from build123d import *

# Parameters (mm, degrees)
ESQUISSE1_W             = 110
ESQUISSE1_H             = 70
BOSS_EXTRU_1_DEPTH      = 5
ESQUISSE2_R             = 2.5
ESQUISSE2_R_2           = 1.3
ENL_V_MAT_EXTRU_1_DEPTH = 131.479883507
ESQUISSE4_R             = 2.5
ENL_V_MAT_EXTRU_2_DEPTH = 3
ENL_V_MAT_EXTRU_3_DEPTH = 131.479883507
CONG_1_R                = 10


with BuildPart() as part:
    # Esquisse1 → Boss.-Extru.1 (new body)
    with BuildSketch(Plane(origin=(0, 0, 0), x_dir=(1, 0, 0), z_dir=(0, 1, 0))):
        with Locations((55, 35)):
            Rectangle(ESQUISSE1_W, ESQUISSE1_H)
    extrude(amount=BOSS_EXTRU_1_DEPTH)

    # Esquisse2 → Enlèv. mat.-Extru.1 (cut, through all)
    with BuildSketch(Plane(origin=(0, 5, 0), x_dir=(1, 0, 0), z_dir=(0, 1, 0))):
        with Locations(Location((9, 59, 0), (0, 0, 270))):
            Circle(ESQUISSE2_R)
        with Locations(Location((9, 11, 0), (0, 0, 270))):
            Circle(ESQUISSE2_R)
        with Locations(Location((101, 11, 0), (0, 0, 270))):
            Circle(ESQUISSE2_R)
        with Locations(Location((101, 59, 0), (0, 0, 270))):
            Circle(ESQUISSE2_R)
        with Locations(Location((25, 46.176778867, 0), (0, 0, 270))):
            Circle(ESQUISSE2_R_2)
        with Locations(Location((25, 21.176778867, 0), (0, 0, 270))):
            Circle(ESQUISSE2_R_2)
        with Locations(Location((85, 21.176778867, 0), (0, 0, 270))):
            Circle(ESQUISSE2_R_2)
        with Locations(Location((85, 46.176778867, 0), (0, 0, 270))):
            Circle(ESQUISSE2_R_2)
    extrude(amount=-ENL_V_MAT_EXTRU_1_DEPTH, mode=Mode.SUBTRACT)

    # Esquisse4 → Enlèv. mat.-Extru.2 (cut)
    with BuildSketch(Plane(origin=(0, 5, 0), x_dir=(1, 0, 0), z_dir=(0, 1, 0))):
        with Locations(Location((25, 46.176778867, 0), (0, 0, 270))):
            Circle(ESQUISSE4_R)
        with Locations(Location((25, 21.176778867, 0), (0, 0, 270))):
            Circle(ESQUISSE4_R)
        with Locations(Location((85, 21.176778867, 0), (0, 0, 270))):
            Circle(ESQUISSE4_R)
        with Locations(Location((85, 46.176778867, 0), (0, 0, 270))):
            Circle(ESQUISSE4_R)
    extrude(amount=-ENL_V_MAT_EXTRU_2_DEPTH, mode=Mode.SUBTRACT)

    # Esquisse5 → Enlèv. mat.-Extru.3 (cut, through all)
    with BuildSketch(Plane(origin=(0, 5, 0), x_dir=(1, 0, 0), z_dir=(0, 1, 0))):
        with BuildLine():
            Line((35.175146904, 65), (74.824853096, 65))
            ThreePointArc((74.824853096, 65), (79.824853096, 60), (74.824853096, 55))
            Line((74.824853096, 55), (35.175146904, 55))
            ThreePointArc((35.175146904, 55), (30.175146904, 60), (35.175146904, 65))
        make_face()
        with BuildLine():
            Line((16.226090532, 40.659734035), (93.773909468, 40.659734035))
            ThreePointArc((93.773909468, 40.659734035), (99.433643503, 35), (93.773909468, 29.340265965))
            Line((93.773909468, 29.340265965), (16.226090532, 29.340265965))
            ThreePointArc((16.226090532, 29.340265965), (10.566356497, 35), (16.226090532, 40.659734035))
        make_face()
        with BuildLine():
            Line((33.566737233, 15), (76.433262767, 15))
            ThreePointArc((76.433262767, 15), (81.433262767, 10), (76.433262767, 5))
            Line((76.433262767, 5), (33.566737233, 5))
            ThreePointArc((33.566737233, 5), (28.566737233, 10), (33.566737233, 15))
        make_face()
    extrude(amount=-ENL_V_MAT_EXTRU_3_DEPTH, mode=Mode.SUBTRACT)

    # Congé1
    cong_1_edges = [part.edges().sort_by_distance(p)[0] for p in [
        (0, 2.5, -70),
        (110, 2.5, -70),
        (110, 2.5, 0),
        (0, 2.5, 0),
    ]]
    fillet(cong_1_edges, radius=CONG_1_R)


solid = part.part
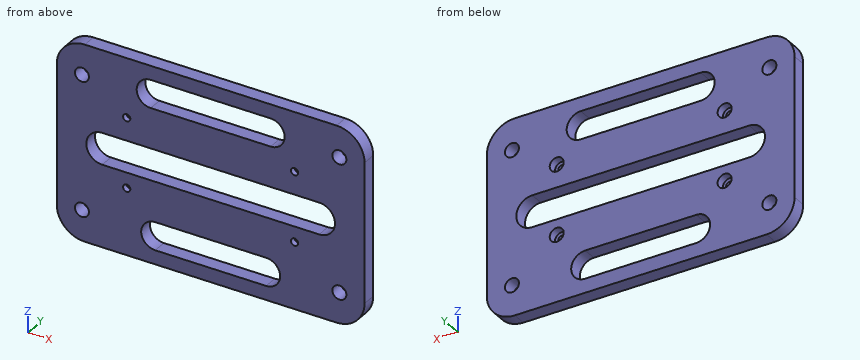
The listing builds one solid part. Answer for the finished solid, in the listing's coordinates (mm). Round coordinates to 2 decimals unless told otherwise and drop trailing zeros. Order: outer loops, then holes, each group sorted by start corner. A loop starts at its lowest first (then second) coordinate and runs counter-clockwise, first axis right, second up. Notation, with made-up numbers: (-6.75, -39) -> (14.25, -39) arc R29 cw to (14.25, -18) -> close; hole circle Ø1 at (-23, -9). An arc over 180 degrees is marked (long way). Write each question's results on one line, items separated by ' | '. Start each with the question number.
Q1. Find section B-B (z = -35). Determine the outline of the cut face in (x, y).
Q2. This flat-tipped pin is pushed along its axis until it touches: pin 1 (5.5 mm diameter, centred on x = 85, z = -20.5, fed in from +Y). Where does it stop, or does it pass through?
Q3. Find section C-C (y = 3.5). Give the number of separate pieces and of enclosed holes in the cut face, then the cut area to 3 significant figures.
Q4. Straight lines are drawn through the part: probe 1 along Z at (x, y) = (66, 4.15); probe 2 along Z at (x, y) = (85, 1.6); probe 3 along X at (y, z) = (1.65, -13). For each, find the intervals that lie inside material, in ascending order. Write a range as from..to.
Q5. Find section A-A (x = 45.5). Determine the outline of the cut face in (y, z), then the cut area to 3 significant figures.
Q6. Find section D-D (x = 25). Determine the outline of the cut face in (y, z).
Worked answers:
1) outline: (0, 0) -> (10.57, 0) -> (10.57, 5) -> (0, 5) -> close; (99.43, 0) -> (110, 0) -> (110, 5) -> (99.43, 5) -> close
2) pin 1: stops at y = 5
3) separate pieces: 1 | enclosed holes: 11 | area: 5,500 mm2
4) probe 1: z = -70..-65, -55..-40.66, -29.34..-15, -5..0 | probe 2: z = -70..-47.48, -44.88..-40.66, -29.34..-22.48, -19.88..0 | probe 3: x = 0..7.5, 10.5..29.57, 80.43..99.5, 102.5..110
5) outline: (0, -70) -> (5, -70) -> (5, -65) -> (0, -65) -> close; (0, -55) -> (5, -55) -> (5, -40.66) -> (0, -40.66) -> close; (0, -29.34) -> (5, -29.34) -> (5, -15) -> (0, -15) -> close; (0, -5) -> (5, -5) -> (5, 0) -> (0, 0) -> close | area: 193 mm2
6) outline: (0, -70) -> (5, -70) -> (5, -48.68) -> (2, -48.68) -> (2, -47.48) -> (0, -47.48) -> close; (0, -44.88) -> (2, -44.88) -> (2, -43.68) -> (5, -43.68) -> (5, -40.66) -> (0, -40.66) -> close; (0, -29.34) -> (5, -29.34) -> (5, -23.68) -> (2, -23.68) -> (2, -22.48) -> (0, -22.48) -> close; (0, -19.88) -> (2, -19.88) -> (2, -18.68) -> (5, -18.68) -> (5, 0) -> (0, 0) -> close
